```python
from build123d import *

# Parameters (mm, degrees)
BOSS_EXTRUDE1_DEPTH      = 1.5
BOSS_EXTRUDE1_DEPTH_BACK = 1.5
BOSS_EXTRUDE2_DEPTH      = 234
FILLET1_R                = 37
FILLET2_R                = 37
FILLET3_R                = 18
FILLET4_R                = 18


with BuildPart() as part:
    # Sketch1 → Boss-Extrude1 (new, two sides: drawn at the far end of the back side and taken through both)
    with BuildSketch(Plane.XY.offset(-BOSS_EXTRUDE1_DEPTH_BACK)):
        Polygon((0, 0), (0, 234), (184, 49), (218, -80), align=None)
    extrude(amount=BOSS_EXTRUDE1_DEPTH + BOSS_EXTRUDE1_DEPTH_BACK)

    # Sketch3 → Boss-Extrude2 (add)
    with BuildSketch(Plane(origin=(0, 0, 0), x_dir=(1, 0, 0), z_dir=(0, 1, 0))):
        with BuildLine():
            Line((0, 0), (0, 20))
            Line((0, 20), (-4.153415616, 20))
            ThreePointArc((-4.153415616, 20), (-1, 0), (-4.153415616, -20))
            Line((-4.153415616, -20), (0, -20))
            Line((0, -20), (0, 0))
        make_face()
    extrude(amount=BOSS_EXTRUDE2_DEPTH)

    # Fillet1
    # the kernel refuses this fillet: 37 mm, written as the material it takes off along each edge
    with BuildSketch(Plane(origin=(0, -42.580944556, -20), x_dir=(-1, 0, 0), z_dir=(0, 1, 0))) as fillet1_piece_1:
        with BuildLine():
            CenterArc((37, 17.032377822), FILLET1_R, 180, 27.408696588)
            Line((0, 17.032377822), (-0.74, 17.032377822))
            Line((-0.74, 17.032377822), (-0.74, 0))
            Line((-0.74, 0), (0, -0.74))
            ThreePointArc((0, -0.74), (2.076707808, -0.74), (3.496483928, -0.340647556))
            Line((3.496483928, -0.340647556), (4.153415616, 0))
        make_face()
    extrude(amount=319.161889112, mode=Mode.SUBTRACT)

    # Fillet2
    # the kernel refuses this fillet: 37 mm, written as the material it takes off along each edge
    with BuildSketch(Plane(origin=(0, -42.580944556, 20), x_dir=(-1, 0, 0), z_dir=(0, 1, 0))) as fillet2_piece_1:
        with BuildLine():
            CenterArc((37, -17.032377822), FILLET2_R, 152.591303412, 27.408696588)
            Line((0, -17.032377822), (-0.74, -17.032377822))
            Line((-0.74, -17.032377822), (-0.74, 0))
            Line((-0.74, 0), (0, 0.74))
            ThreePointArc((0, 0.74), (2.076707808, 0.74), (3.496483928, 0.340647556))
            Line((3.496483928, 0.340647556), (4.153415616, 0))
        make_face()
    extrude(amount=319.161889112, mode=Mode.SUBTRACT)

    # Fillet3
    # the kernel refuses this fillet: 18 mm, written as the material it adds along each edge
    with BuildSketch(Plane(origin=(0, -38.641156858, 1.5), x_dir=(-0.13467815592130583, 0, 0.990889395602575), z_dir=(0, 1, 0))) as fillet3_piece_1_section:
        with BuildLine():
            CenterArc((15.754361222, 17.739851832), FILLET3_R, 187.740009623, 72.507035508)
            Line((-2.081647899, 15.315645026), (-3.865248811, 15.073224345))
            Line((-3.865248811, 15.073224345), (-1.783600912, -0.242420681))
            Line((-1.783600912, -0.242420681), (0.242420681, -1.783600912))
            ThreePointArc((0.242420681, -1.783600912), (1.696671933, -1.585944264), (12.40023467, -1.773985183))
            Line((12.40023467, -1.773985183), (12.705155265, 0))
        make_face()
    fillet3_piece_1 = extrude(amount=272.641156858, mode=Mode.PRIVATE)
    fillet3_piece_1 = fillet3_piece_1 - Plane(origin=(-66, -0.945349387, 0), x_dir=(0.9514859136040758, 0, -0.3076923076923073), z_dir=(0, -1, 0)) * Cylinder(65, 607, mode=Mode.PRIVATE)
    fillet3_piece_1 = split(fillet3_piece_1, bisect_by=Plane(origin=(6.079958866, -2.231177565, 3.815463773), z_dir=(0.34450770303612605, 0.9387834907734437, 0)), keep=Keep.TOP, mode=Mode.PRIVATE)
    fillet3_piece_1 = split(fillet3_piece_1, bisect_by=Plane(origin=(120.729104933, 112.614758628, 3.815463773), z_dir=(-0.7090204561204898, -0.7051879131144355, 0)), keep=Keep.TOP, mode=Mode.PRIVATE)
    add(fillet3_piece_1)
    with BuildSketch(Plane(origin=(0, 0, 1.5), x_dir=(-0.1346781559213058, 0, 0.990889395602575), z_dir=(0, 1, 0))) as fillet3_piece_2_section:
        with BuildLine():
            CenterArc((15.754361222, 17.739851832), FILLET3_R, 187.740009623, 72.507035508)
            Line((-2.081647899, 15.315645026), (-3.865248811, 15.073224345))
            Line((-3.865248811, 15.073224345), (-1.783600912, -0.242420681))
            Line((-1.783600912, -0.242420681), (0.242420681, -1.783600912))
            ThreePointArc((0.242420681, -1.783600912), (1.696671933, -1.585944264), (12.40023467, -1.773985183))
            Line((12.40023467, -1.773985183), (12.705155265, 0))
        make_face()
    fillet3_piece_2 = extrude(amount=272.641156858, mode=Mode.PRIVATE)
    fillet3_piece_2 = fillet3_piece_2 - Plane(origin=(-66, 0.313964565, 0), x_dir=(0.9514859136040758, 0, -0.3076923076923073), z_dir=(0, -1, 0)) * Cylinder(65, 607, mode=Mode.PRIVATE)
    fillet3_piece_2 = split(fillet3_piece_2, bisect_by=Plane(origin=(-0.982422038, 0.360521849, 12.117700452), z_dir=(-0.34450770303612605, -0.9387834907734437, 0)), keep=Keep.TOP, mode=Mode.PRIVATE)
    add(fillet3_piece_2)

    # Fillet4
    # the kernel refuses this fillet: 18 mm, written as the material it adds along each edge
    with BuildSketch(Plane(origin=(0, -38.641156858, -1.5), x_dir=(-0.1346781559213057, 0, -0.990889395602575), z_dir=(0, 1, 0))) as fillet4_piece_1_section:
        with BuildLine():
            CenterArc((15.754361222, -17.739851832), FILLET4_R, 99.752954869, 72.507035508)
            Line((-2.081647899, -15.315645026), (-3.865248811, -15.073224345))
            Line((-3.865248811, -15.073224345), (-1.783600912, 0.242420681))
            Line((-1.783600912, 0.242420681), (0.242420681, 1.783600912))
            ThreePointArc((0.242420681, 1.783600912), (1.696671933, 1.585944264), (12.40023467, 1.773985183))
            Line((12.40023467, 1.773985183), (12.705155265, 0))
        make_face()
    fillet4_piece_1 = extrude(amount=272.641156858, mode=Mode.PRIVATE)
    fillet4_piece_1 = fillet4_piece_1 - Plane(origin=(-66, -0.945349387, 0), x_dir=(0.9514859136040758, 0, -0.3076923076923073), z_dir=(0, -1, 0)) * Cylinder(65, 607, mode=Mode.PRIVATE)
    fillet4_piece_1 = split(fillet4_piece_1, bisect_by=Plane(origin=(120.729104933, 112.614758628, -3.815463773), z_dir=(-0.709020456120464, -0.7051879131144615, 0)), keep=Keep.TOP, mode=Mode.PRIVATE)
    fillet4_piece_1 = split(fillet4_piece_1, bisect_by=Plane(origin=(6.079958866, -2.231177565, -3.815463773), z_dir=(0.34450770303615846, 0.9387834907734318, 0)), keep=Keep.TOP, mode=Mode.PRIVATE)
    add(fillet4_piece_1)
    with BuildSketch(Plane(origin=(0, 0, -1.5), x_dir=(-0.13467815592130572, 0, -0.990889395602575), z_dir=(0, 1, 0))) as fillet4_piece_2_section:
        with BuildLine():
            CenterArc((15.754361222, -17.739851832), FILLET4_R, 99.752954869, 72.507035508)
            Line((-2.081647899, -15.315645026), (-3.865248811, -15.073224345))
            Line((-3.865248811, -15.073224345), (-1.783600912, 0.242420681))
            Line((-1.783600912, 0.242420681), (0.242420681, 1.783600912))
            ThreePointArc((0.242420681, 1.783600912), (1.696671933, 1.585944264), (12.40023467, 1.773985183))
            Line((12.40023467, 1.773985183), (12.705155265, 0))
        make_face()
    fillet4_piece_2 = extrude(amount=272.641156858, mode=Mode.PRIVATE)
    fillet4_piece_2 = fillet4_piece_2 - Plane(origin=(-66, 0.313964565, 0), x_dir=(0.9514859136040758, 0, -0.3076923076923073), z_dir=(0, -1, 0)) * Cylinder(65, 607, mode=Mode.PRIVATE)
    fillet4_piece_2 = split(fillet4_piece_2, bisect_by=Plane(origin=(-0.982422038, 0.360521849, -12.117700452), z_dir=(-0.34450770303615846, -0.9387834907734318, 0)), keep=Keep.TOP, mode=Mode.PRIVATE)
    add(fillet4_piece_2)


solid = part.part
```
The listing builds one solid part. Answer for the finished solid, in the listing's coordinates (mm). A direction names the side the tool comes from. Coordinates: 2 decimals unless noted, no trailing zeros. Loops run counter-clockwise (first coordinate to the right, second up) from the corner with the lowest first, then second, coordinate; pieces in that order, holes last. Notation, with made-up numbers: M 72,45 L 123,45 A8 ccw 123,50 Z; hole C 37.25,26.25 d2. An arc over 180 degrees is marked long. Answer as a JSON object with one key per item and string values. Group by question number.
Item 1: Which of the six approach directions +Z, -Z, +X, -X, +Y, -Y give full straight-line access (tool end or side, diameter ignored) to faces 1 (the face through (77.941, 155.635, 0.048)), 2 (the face through (96, 38, -1.5)), 3 (the face through (96, 38, 1.5))?
Item 2: Section D-D (x = 125) is taken. Write down the section's boundary in (y, z).
Item 3: Section A-A (y = 192.5) is taken. Write down the section's boundary in (x, z).
Item 4: Section B-B (x = 200.5) is taken. Write down the section's boundary in (y, z), and give its area (3 significant figures).
Item 5: Section C-C (y = 91) is taken. Write down the section's boundary in (x, z).
Item 6: Consider L1, parallel to Z at x = 114, y = -13; L2, parallel to Z at x = 5, y = 132; L3, parallel to X at y = 46, z = -3. Determine where each line is inside the solid, lowest interval first.
Item 7: Each of these flat-tipped pins is pushed along its axis until it touches: P1, Ø5, axis at y = 68.5, z = 9.5, coming from the +X side; P2, Ø12, axis at x = 52, z = 3, coming from the -Y side; P3, Ø1.5, axis at y = 1.5, z = -7, coming from the -X side. Where does it stop, or does it pass through?
Solved:
{
 "1": {"face 1": "+Z, -Z, +X, +Y", "face 2": "-Z, +X, +Y, -Y", "face 3": "+Z, +X, +Y, -Y"},
 "2": {"outline": "M -45.87,-1.5 L 108.32,-1.5 L 108.32,1.5 L -45.87,1.5 Z"},
 "3": {"outline": "M -4.15,-20 A37 ccw -1.71,-14.09 A18 cw 15.46,-1.5 L 41.28,-1.5 L 41.28,1.5 L 15.46,1.5 A18 cw -1.71,14.09 A37 ccw -4.15,20 A65 cw Z"},
 "4": {"outline": "M -73.58,-1.5 L -13.6,-1.5 L -13.6,1.5 L -73.58,1.5 Z", "area": "180 mm2"},
 "5": {"outline": "M -4.15,-20 A37 ccw -1.71,-14.09 A18 cw 15.46,-1.5 L 142.23,-1.5 L 142.23,1.5 L 15.46,1.5 A18 cw -1.71,14.09 A37 ccw -4.15,20 A65 cw Z"},
 "6": {"L1": "z = -1.5 to 1.5", "L2": "z = -4.85 to 4.85", "L3": "x = -1.07 to 8.26"},
 "7": {"P1": "stops at x = 2.5", "P2": "stops at y = -21.21", "P3": "stops at x = -1.46"}
}
